from build123d import *

# Parameters (mm, degrees)
F1_DEPTH = 25.4
F2_R     = 5.08
F3_R     = 5.08
F4_R     = 5.08
F5_R     = 5.08


with BuildPart() as f1:
    # F0 (on Top) → F1 (new body)
    with BuildSketch(Plane.XY):
        Polygon((0, 50.8), (0, 0), (152.4, 0), (152.4, 76.2), (101.6, 76.2), (101.6, 50.8), align=None)
    extrude(amount=-F1_DEPTH)

    # F2
    f2_edges = [f1.edges().sort_by_distance(p)[0] for p in [
        (152.4, 76.2, -12.7),
    ]]
    fillet(f2_edges, radius=F2_R)

    # F3
    f3_edges = [f1.edges().sort_by_distance(p)[0] for p in [
        (0, 50.8, -12.7),
    ]]
    fillet(f3_edges, radius=F3_R)

    # F4
    f4_edges = [f1.edges().sort_by_distance(p)[0] for p in [
        (0, 0, -12.7),
    ]]
    fillet(f4_edges, radius=F4_R)

    # F5
    f5_edges = [f1.edges().sort_by_distance(p)[0] for p in [
        (152.4, 0, -12.7),
    ]]
    fillet(f5_edges, radius=F5_R)


solid = f1.part
The listing builds one solid part. Answer for the finished solid, in the listing's coordinates (mm). A direction names the side the tool comes from. Round coordinates to 2 decimals unless told otherwise and drop trailing zeros. Loops run counter-clockwise (first coordinate to the right, second up) from the corner with the lowest first, then second, coordinate; pieces in that order, holes last. Notation, with made-up numbers: M 43.5,68 L 97.5,68 A22 cw 97.5,106 Z; hole C -4.5,37 d7. An arc over 180 degrees is marked long. Return JSON: item names as keys, results as strings.
Q1. Find section A-A, the plane z = -9.5. Determine the outline of the cut face in (x, y), plus the area to 3 significant figures.
Results list:
{"outline": "M 0,5.08 A5.08 ccw 5.08,0 L 147.32,0 A5.08 ccw 152.4,5.08 L 152.4,71.12 A5.08 ccw 147.32,76.2 L 101.6,76.2 L 101.6,50.8 L 5.08,50.8 A5.08 ccw 0,45.72 Z", "area": "9,010 mm2"}
Q2. Each of these flat-tipped pins is pushed along its axis until it touches: pin 1 Ø8 at (y, z) = (65.5, -12) entering from -X; pin 2 Ø7.5 at (x, z) = (67, -13.5) entering from +Y. Where does it stop, or does it pass through?
Results list:
{"pin 1": "stops at x = 101.6", "pin 2": "stops at y = 50.8"}
Q3. Find section B-B, the plane x = 61. Determine the outline of the cut face in (y, z).
Results list:
{"outline": "M 0,-25.4 L 50.8,-25.4 L 50.8,0 L 0,0 Z"}
Q4. Find section C-C, the plane y = 55.5. Determine the outline of the cut face in (x, z), plus the area to 3 significant figures.
Results list:
{"outline": "M 101.6,-25.4 L 152.4,-25.4 L 152.4,0 L 101.6,0 Z", "area": "1,290 mm2"}
Q5. Which of the six approach directions +Z, -Z, +X, -X, +Y, -Y give full straight-line access (tool end or side, diameter ignored) to faces 1 (the face through (75, 0, -13)), 2 (the face through (101.6, 64, -13))?
Results list:
{"face 1": "+Z, -Z, +X, -X, -Y", "face 2": "+Z, -Z, -X, +Y"}
Q6. Find the intervals of material crossed by line 1 along Y through (x, z) = (72, -21.25); line 2 along X through (y, z) = (71.5, -5); line 3 along X through (y, z) = (72, -6), in increasing order. Write a range as from..to.
Results list:
{"line 1": "y = 0..50.8", "line 2": "x = 101.6..152.39", "line 3": "x = 101.6..152.32"}
